For this review, use the dimensioned drawing (mm, ordinates from the lowest corner) and the shaded views. Round coordinates to 2 decimals unless told otherwise and drop trailing zeros. Order: outer loops, then holes, each group sorted by start corner. A loop starts at its lowest first (then second) coordinate and runs counter-clockwise, first axis right, second up. Notation, with made-up numbers: (35.5, 66) -> (74.5, 66) arc R21 cw to (74.5, 82) -> close; hole circle Ø5 at (-6, 21.25). An arc over 180 degrees is marked (long way). Answer in a Markdown table with one row per item.
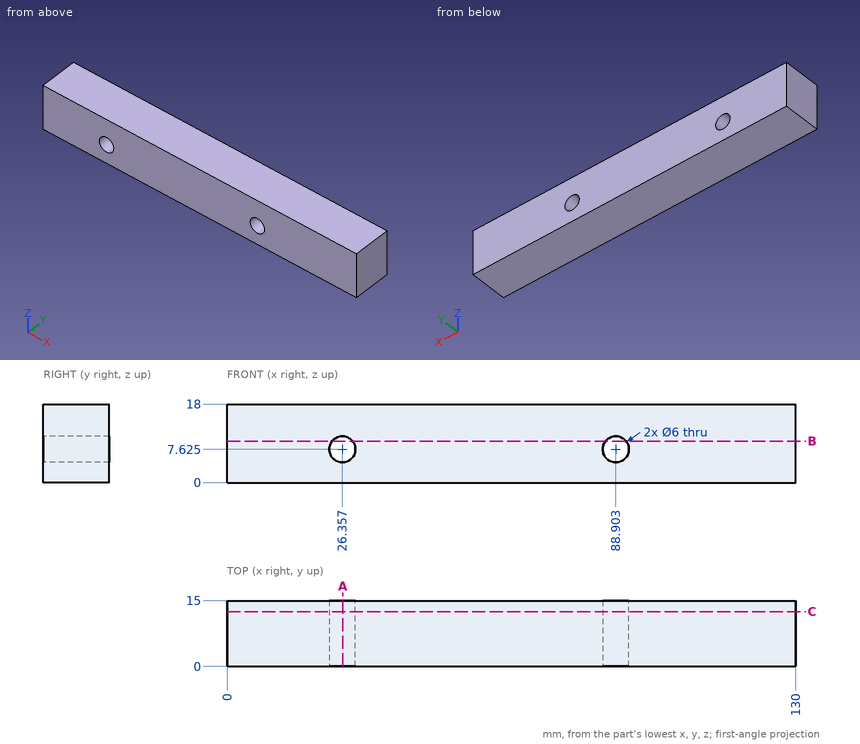
Q1. Take a section at C-C, the plane y = 12.5. Write out the cut boundary in (x, z) (1 decimal).
Answer key:
| item | result |
|---|---|
| outline | (0, 0) -> (130, 0) -> (130, 18) -> (0, 18) -> close; hole circle Ø6 at (26.4, 7.6); hole circle Ø6 at (88.9, 7.6) |
Q2. Take a section at B-B, the plane z = 9.5. Write out the cut boundary in (x, y) (1 decimal), then the cut area to 3 significant figures.
Answer key:
| item | result |
|---|---|
| outline | (0, 0) -> (24, 0) -> (24, 15) -> (0, 15) -> close; (28.7, 0) -> (86.6, 0) -> (86.6, 15) -> (28.7, 15) -> close; (91.2, 0) -> (130, 0) -> (130, 15) -> (91.2, 15) -> close |
| area | 1,810 mm^2 |
Q3. Take a section at A-A, the plane x = 26.5. Write out the cut boundary in (y, z).
Answer key:
| item | result |
|---|---|
| outline | (0, 0) -> (15, 0) -> (15, 4.63) -> (0, 4.63) -> close; (0, 10.62) -> (15, 10.62) -> (15, 18) -> (0, 18) -> close |
Q4. To check wall thickness, follow probe 1 along X at (y, z) = (9.5, 6.25) (1 decimal); probe 2 along X at (y, z) = (2.5, 5.5) (1 decimal). State the ranges of each line that lie inside material, in increasing order.
Answer key:
| item | result |
|---|---|
| probe 1 | x = 0 to 23.7, 29 to 86.2, 91.6 to 130 |
| probe 2 | x = 0 to 24.2, 28.5 to 86.8, 91 to 130 |
